```python
from build123d import *

# Parameters (mm, degrees)
BOSS_EXTRUDE1_DEPTH   = 7.25
SKETCH2_W             = 2.5
SKETCH2_H             = 3
BOSS_EXTRUDE2_DEPTH   = 8.25
BOSS_EXTRUDE2_2_DEPTH = 8.25
BOSS_EXTRUDE2_3_DEPTH = 8.25
BOSS_EXTRUDE2_4_DEPTH = 8.25
SKETCH3_W             = 3
SKETCH3_H             = 3.25
BOSS_EXTRUDE3_DEPTH   = 1.5


with BuildPart() as part:
    # Sketch1 → Boss-Extrude1 (new body)
    with BuildSketch(Plane.XY):
        Polygon((-4.25, 58.75), (8.25, 58.75), (8.25, 55.5), (11.25, 55.5), (11.25, 58.75), (27.75, 58.75), (27.75, 55.5), (30.75, 55.5), (30.75, 58.75), (33.5, 58.75), (33.5, 52.5), (24.75, 52.5), (24.75, 55.75), (14.25, 55.75), (14.25, 52.5), (5.25, 52.5), (5.25, 55.75), (-1.25, 55.75), (-1.25, -5.25), (5.25, -5.25), (5.25, -2), (14.25, -2), (14.25, -5.25), (24.75, -5.25), (24.75, -2), (33.5, -2), (33.5, -8.25), (30.75, -8.25), (30.75, -5), (27.75, -5), (27.75, -8.25), (11.25, -8.25), (11.25, -5), (8.25, -5), (8.25, -8.25), (-4.25, -8.25), align=None)
    extrude(amount=BOSS_EXTRUDE1_DEPTH)



with BuildPart() as body_2:
    # Sketch2 → Boss-Extrude2 (new body)
    with BuildSketch(Plane.XY.offset(5.75)):
        with Locations((9.75, -6.75)):
            Rectangle(SKETCH2_W, SKETCH2_H)
    extrude(amount=BOSS_EXTRUDE2_DEPTH)


with BuildPart() as body_3:
    # Sketch2 → Boss-Extrude2 2 (new body)
    with BuildSketch(Plane.XY.offset(5.75)):
        with Locations((29.25, -6.75)):
            Rectangle(SKETCH2_W, SKETCH2_H)
    extrude(amount=BOSS_EXTRUDE2_2_DEPTH)


with BuildPart() as body_4:
    # Sketch2 → Boss-Extrude2 3 (new body)
    with BuildSketch(Plane.XY.offset(5.75)):
        with Locations((29.25, 57.25)):
            Rectangle(SKETCH2_W, SKETCH2_H)
    extrude(amount=BOSS_EXTRUDE2_3_DEPTH)


with BuildPart() as body_5:
    # Sketch2 → Boss-Extrude2 4 (new body)
    with BuildSketch(Plane.XY.offset(5.75)):
        with Locations((9.75, 57.25)):
            Rectangle(SKETCH2_W, SKETCH2_H)
    extrude(amount=BOSS_EXTRUDE2_4_DEPTH)


with BuildPart() as part_1:
    add(part.part)

    add(body_2.part)  # Boss-Extrude3 merges body 2

    add(body_3.part)  # Boss-Extrude3 merges body 3

    add(body_4.part)  # Boss-Extrude3 merges body 4

    add(body_5.part)  # Boss-Extrude3 merges body 5
    # Sketch3 → Boss-Extrude3 (add)
    with BuildSketch(Plane(origin=(0, 0, 5.75), x_dir=(-1, 0, 0), z_dir=(0, 0, -1))):
        with Locations((-9.75, 57.125)):
            Rectangle(SKETCH3_W, SKETCH3_H)
        with Locations((-29.25, 57.125)):
            Rectangle(SKETCH3_W, SKETCH3_H)
        with Locations((-29.25, -6.625)):
            Rectangle(SKETCH3_W, SKETCH3_H)
        with Locations((-9.75, -6.625)):
            Rectangle(SKETCH3_W, SKETCH3_H)
    extrude(amount=-BOSS_EXTRUDE3_DEPTH)


solid = part_1.part
```
Design review of the part built by this model. Coordinates are the model's own, in mm. A direction names the side the tool comes from. Coordinates: 2 decimals unless noted, no trailing zeros. Write each loop counter-clockwise with the first axis right and the second up, starting at its lowest first coordinate (ties: lowest second). Pieces come first, ordered by that corner, then holes.
1) Add section A-A (z = 8.25). Write out the cut boundary in (x, y).
2) Add section D-D (y = 6.5). Write out the cut boundary in (x, z).
3) Mouldability with a two-part tool opening along X and no side actions: class faces 1 (the flat face through (24.75, 54, 4)), 2 (the flat face through (10, -7, 14)), 3 (the flat face through (-4.25, 25, 4)), 4 (the flat face through (33.5, -5, 4)) as +X half, -X half, draft (parallel to the pull), parting line (faces both ways), or undercut.
4) Add section C-C (x = 3). Write out the cut boundary in (y, z), plus the area to 3 significant figures.
5) To check wall thickness, follow L1, parallel to X at y = 53.5, z = 3; L2, parallel to Y at x = 20.5, z = 4; L3, parallel to Y at x = 32.5, z = 5.25. State the ranges of each line that lie inside material, in increasing order.
6) Insertion check: pin 1 (0.9 mm diameter, centred on x = 9.5, y = 56.5, fed in from -Z); pin 2 (8 mm diameter, centred on x = 0.5, y = 20.5, fed in from +Z); pin 3 (0.9 mm diameter, centred on x = 10, z = 2, fed in from -Y). Each pin has a flat end and moves straight along its axis. Give the tip position at first contact, or say it passes through.
7) Add section B-B (x = 9.5). Write out the cut boundary in (y, z), plus the area to 4 significant figures.
8) Machinability: for faces 5 (the flat face through (8.25, -7, 3)), 6 (the flat face through (10, 55.5, 3)), 7 (the flat face through (29, 55.75, 11)), 8 (the flat face through (24.75, -4, 4)), which of the approach directions +Z, -Z, +X, -X, +Y, -Y give a long, thin tool a straight path to every point of the face, cutting with its end or side? Answer none if there is none.
Check result:
1. outline: (8.5, -8.25) - (11, -8.25) - (11, -5.25) - (8.5, -5.25) - close; (8.5, 55.75) - (11, 55.75) - (11, 58.75) - (8.5, 58.75) - close; (28, -8.25) - (30.5, -8.25) - (30.5, -5.25) - (28, -5.25) - close; (28, 55.75) - (30.5, 55.75) - (30.5, 58.75) - (28, 58.75) - close
2. outline: (-4.25, 0) - (-1.25, 0) - (-1.25, 7.25) - (-4.25, 7.25) - close
3. face 1: undercut
3. face 2: draft
3. face 3: -X half
3. face 4: +X half
4. outline: (-8.25, 0) - (-5.25, 0) - (-5.25, 7.25) - (-8.25, 7.25) - close; (55.75, 0) - (58.75, 0) - (58.75, 7.25) - (55.75, 7.25) - close
4. area: 43.5 mm2
5. L1: x = -4.25 to -1.25, 5.25 to 14.25, 24.75 to 33.5
5. L2: y = -8.25 to -5.25, 55.75 to 58.75
5. L3: y = -8.25 to -2, 52.5 to 58.75
6. pin 1: stops at z = 5.75
6. pin 2: stops at z = 7.25
6. pin 3: stops at y = -5
7. outline: (-8.25, 5.75) - (-5, 5.75) - (-5, 0) - (-2, 0) - (-2, 7.25) - (-5.25, 7.25) - (-5.25, 14) - (-8.25, 14) - close; (52.5, 0) - (55.5, 0) - (55.5, 5.75) - (58.75, 5.75) - (58.75, 14) - (55.75, 14) - (55.75, 7.25) - (52.5, 7.25) - close
7. area: 93.75 mm2
8. face 5: -Z, -Y
8. face 6: -Z, +Y
8. face 7: +Z, +X, -X
8. face 8: +Z, -Z
